Input: dimensioned drawing with shaded views. Units: mm. Origin: part minimum x, y, z. Give positions to 0.01 mm unless a question says otherwise; leave off trailing zeros. Order: outer loops, then holes, each group sorted by start corner. A loop starts at its lowest first (then second) coordinate and runs counter-clockwise, first axis right, second up. Notation, with made-up numbers: (40.25, -4.75) -> (59.25, -4.75) arc R8 ccw to (59.25, -0.75) -> close; hole circle Ø3 at (-20.5, 53). An arc over 180 degrees is marked (long way). Use CSV: the item, a comma, the result in double quotes.
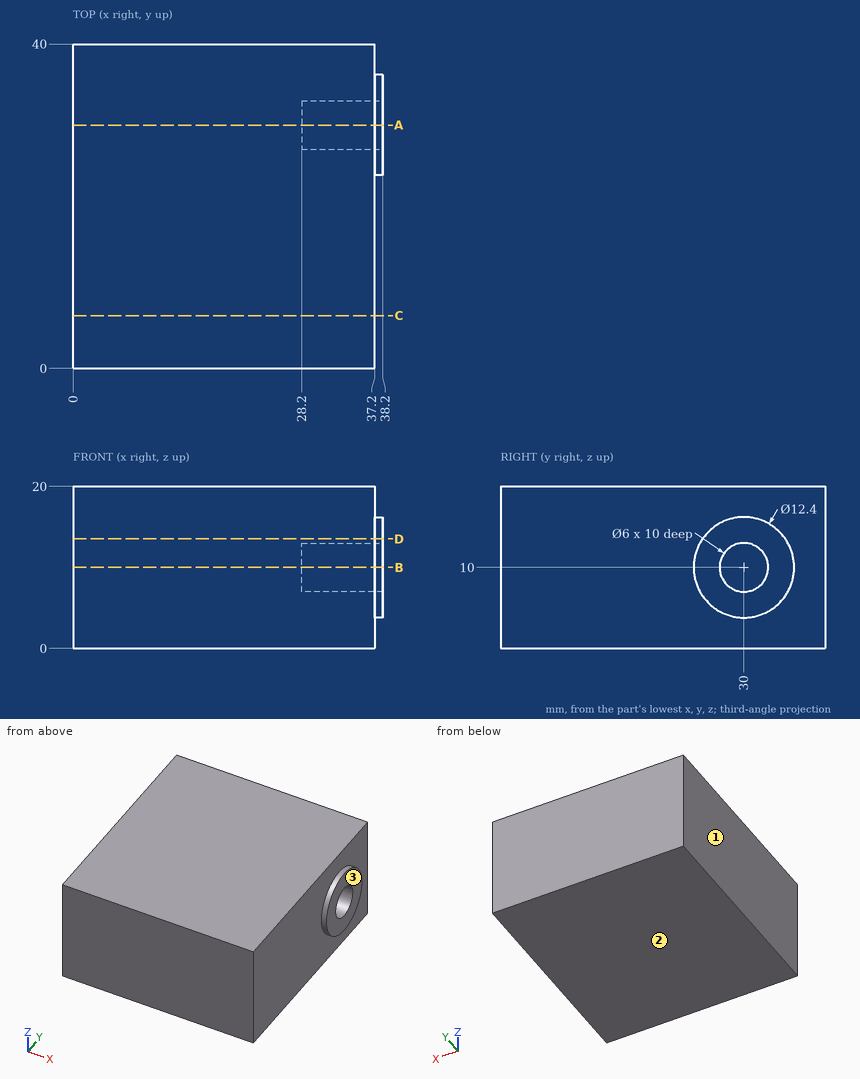
1. Section query B-B on z = 10. Return loops of the section in (x, y), plus the area to 3 significant figures.
Answer below:
outline,"(0, 0) -> (37.2, 0) -> (37.2, 23.8) -> (38.2, 23.8) -> (38.2, 27) -> (28.2, 27) -> (28.2, 33) -> (38.2, 33) -> (38.2, 36.2) -> (37.2, 36.2) -> (37.2, 40) -> (0, 40) -> close"
area,"1,440 mm²"
2. Mould query, pull axis X, two halves, no side actions, for the marked faces 1, 2 and 3. Classes: released by +X, released by -X, zero draft, split by the parting line, or undercut.
Answer below:
face 1,"released by -X"
face 2,"zero draft"
face 3,"released by +X"
3. Section query C-C on y = 6.5. Return loops of the section in (x, z).
Answer below:
outline,"(0, 0) -> (37.2, 0) -> (37.2, 20) -> (0, 20) -> close"
4. Section query A-A on y = 30. Return loops of the section in (x, z).
Answer below:
outline,"(0, 0) -> (37.2, 0) -> (37.2, 3.8) -> (38.2, 3.8) -> (38.2, 7) -> (28.2, 7) -> (28.2, 13) -> (38.2, 13) -> (38.2, 16.2) -> (37.2, 16.2) -> (37.2, 20) -> (0, 20) -> close"
5. Pin query (flat end, axial travel): P1, Ø6.5, axis at y = 29, z = 9.5, coming from the +X side. Return the tip coordinate at first contact, or that it passes through.
Answer below:
P1,"stops at x = 38.2"
6. Ray query, line 1 along Y through (x, z) = (33.75, 10); line 2 along X through (y, z) = (15, 4.5); line 3 along X through (y, z) = (29.5, 8). Return the intervals inside material, ascending.
Answer below:
line 1,"y = 0 to 27, 33 to 40"
line 2,"x = 0 to 37.2"
line 3,"x = 0 to 28.2"
7. Section query D-D on z = 13.5. Return loops of the section in (x, y), plus the area to 3 significant figures.
Answer below:
outline,"(0, 0) -> (37.2, 0) -> (37.2, 24.88) -> (38.2, 24.88) -> (38.2, 35.12) -> (37.2, 35.12) -> (37.2, 40) -> (0, 40) -> close"
area,"1,500 mm²"
